Build history of the part. All positions in model axes, mm. Round coordinates to 2 decimals unless told otherwise and drop trailing zeros. Write each loop counter-clockwise with the first axis right and the second up, starting at its lowest first coordinate (ties: lowest second). Pieces come first, ordered by that corner, then holes. Notation, with made-up numbers: M 50.5,59.25 L 73.5,59.25 A13 ccw 73.5,64.25 Z; hole C -22,-31.5 d1. An arc over 180 degrees is marked long. One line per item, written item: value. Start each with the question number.
Autodesk Inventor part; units mm, degrees
ref_plane "YZ Plane" through (0, 0, 0) normal (1, 0, 0) x (0, 1, 0)
ref_plane "XZ Plane" through (0, 0, 0) normal (0, 1, 0) x (-1, 0, 0)
ref_plane "XY Plane" through (0, 0, 0) normal (0, 0, 1) x (1, 0, 0)
sketch "Sketch1" plane through (0, 0, 0) normal (0, 1, 0) x (-1, 0, 0)
  circle A0 centre (50.0013, 74.8323) radius 1.6
  circle A1 centre (-50.0013, 74.8323) radius 1.6
  circle A2 centre (-88.2707, 17.5581) radius 1.6
  circle A3 centre (88.2707, 17.5581) radius 1.6
  line L0 (0, 0) -> (89.861, 0)
  line L1 (0, 0) -> (-89.861, 0)
  arc A4 (94.8533, 5.2778) -> (-94.8533, 5.2778) centre (0, 0) ccw
  arc A5 (89.861, 0) -> (94.8533, 5.2778) centre (89.861, 5) ccw
  arc A6 (-94.8533, 5.2778) -> (-89.861, 0) centre (-89.861, 5) ccw
  point P0 (95, 0)
  point P1 (-95, 0)
  dimension "d39" = 3.2
  dimension "d40" = 3.2
  dimension "d41" = 3.2
  dimension "d43" = 5
extrude "Extrusion1" add sketch "Sketch1" along normal blind 3
properties part number "Top Plate"
Item 1: Cut at A-A, the plane y = 0.95. Write the cut outline in (x, z), plus the area to 3 significant figures.
Item 2: Cut at B-B, the plane x = -41. Write the cut outline in (y, z).
Item 3: Two-plate mould, pull along Z, no slides. Class faces 1 (the cylindrical face through (89.87, 1.48, 17.49)), 2 (the flat face through (1, 3, 38)), 3 (the cylindrical face through (48.475, 1.479, 74.352)), 4 (the cylindrical face through (2.02, 1.48, 94.98)): pulls with the +Z half, pulls with the -Z half, needs draft (parallel to the pull), parting line crosses it, or undercut.
Item 4: Drop a flat-ended pin along its axis: pin 1 (2.5 mm diameter, centred on x = -50, z = 74.83, fed in from +Y). Give the stop position or say it passes through.
Item 5: Cut at C-C, the plane x = 73.5. Write the cut outline in (y, z).
Item 6: Drill centre lines: line 1 (X direction, y = 0.25, z = 17.5); line 2 (X direction, y = 2.3, z = 18); line 3 (Z direction, x = 69, y = 0.6). Where is each one in solid material? Low to high.
Computed values:
1. outline: M -94.85,5.28 A5 ccw -89.86,0 L 89.86,0 A5 ccw 94.85,5.28 A95 ccw Z; hole C -88.27,17.56 d3.2; hole C -50,74.83 d3.2; hole C 50,74.83 d3.2; hole C 88.27,17.56 d3.2
1. area: 14,100 mm2
2. outline: M 0,0 L 3,0 L 3,85.7 L 0,85.7 Z
3. face 1: undercut
3. face 2: needs draft
3. face 3: undercut
3. face 4: pulls with the +Z half
4. pin 1: passes through
5. outline: M 0,0 L 3,0 L 3,60.19 L 0,60.19 Z
6. line 1: x = -93.37 to -89.87, -86.67 to 86.67, 89.87 to 93.37
6. line 2: x = -93.28 to -89.81, -86.73 to 86.73, 89.81 to 93.28
6. line 3: z = 0 to 65.3
